Job drawing, mm, ordinate dimensions from the low corner. One solid piece. A direction names the side the tool comes from. Round coordinates to 2 decimals unless told otherwise and drop trailing zeros. Write each loop counter-clockwise with the first axis right and the second up, starting at its lowest first coordinate (ties: lowest second). Pieces come first, ordered by that corner, then holes. Notation, with made-up numbers: (1.25, -20.5) -> (51.25, -20.5) arc R20 cw to (51.25, 2.5) -> close; hole circle Ø6 at (-26.75, 3). An arc over 180 degrees is marked (long way). Use CSV: the item, a comma, the result in double quotes. Start each with the question number.
(1) Which spindle directions (+Z, -Z, +X, -X, +Y, -Y) get a long thin tool onto all of the face, cutting with end or side? Do the marked faces 4 and 5. Say none if no direction does.
(2) Saw through at C-C (x = 67.5). Give the cut face in (y, z).
(3) Probe line 1 (X direction, y = 4, z = 127); line 2 (X direction, y = 10.25, z = 24.5); line 3 (Z direction, x = 27, y = 0.5). List the from-to ranges inside material, lowest first. Write a range as [from, to].
(4) Drop flat-ended pins along their axis: pin 1 (1.5 mm diameter, centred on y = 1.5, z = 72, fed in from +X) (1 decimal); pin 2 (5 mm diameter, centred on x = 51.5, z = 98.5, fed in from -Y); pin 3 (3 mm diameter, centred on x = 62, y = 10.5, fed in from -Z); pin 4 (3 mm diameter, centred on x = 75, y = 2.5, fed in from -Z) (1 decimal). Give the stop position or say it passes through.
(5) Saw through at B-B (z = 113.5). Give the cut face in (x, y), plus the area to 3 significant figures.
(6) Saw through at A-A (y = 6.5). Give the cut face in (x, z).
(7) Two-plate mould, pull along Z, no slides. Class the marked faces 1, 2 and 3: released by +Z, released by -Z, zero draft, split by the parting line, or undercut.
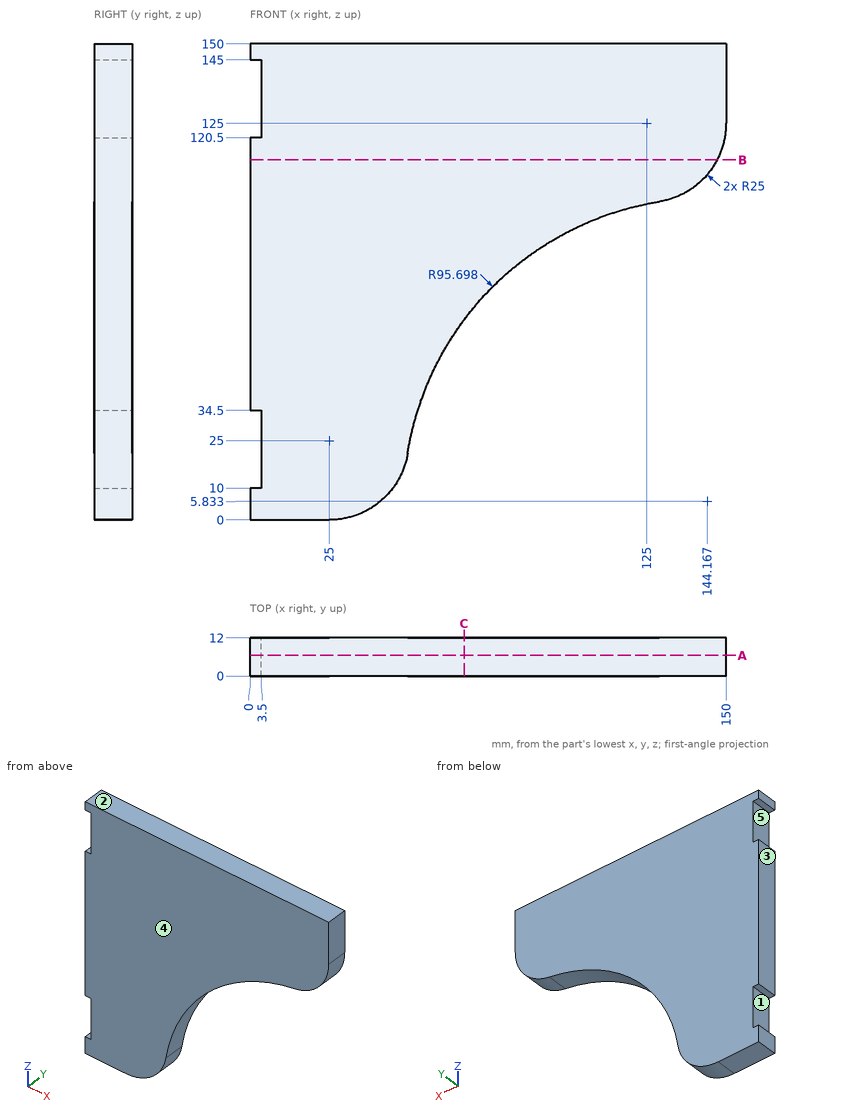
Answers:
1,face 4,"+Z, -Z, +X, -X, -Y"
1,face 5,"-X, +Y, -Y"
2,outline,"(0, 63.11) -> (12, 63.11) -> (12, 150) -> (0, 150) -> close"
3,line 1,"x = [3.5, 150]"
3,line 2,"x = [3.5, 50.31]"
3,line 3,"z = [0.08, 150]"
4,pin 1,"stops at x = 75.8"
4,pin 2,"stops at y = 0"
4,pin 3,"stops at z = 52.29"
4,pin 4,"stops at z = 70.4"
5,outline,"(0, 0) -> (147.2, 0) -> (147.2, 12) -> (0, 12) -> close"
5,area,"1,770 mm²"
6,outline,"(0, 0) -> (25, 0) arc R25 ccw to (49.68, 21.03) arc R95.7 cw to (128.97, 100.32) arc R25 ccw to (150, 125) -> (150, 150) -> (0, 150) -> (0, 145) -> (3.5, 145) -> (3.5, 120.5) -> (0, 120.5) -> (0, 34.5) -> (3.5, 34.5) -> (3.5, 10) -> (0, 10) -> close"
7,face 1,"undercut"
7,face 2,"released by +Z"
7,face 3,"zero draft"
